Here's the drawing with two shaded views (mm, measured from the low corner). I have some questions. A direction names the side the tool comes from. Give positions to 0.01 mm unless a question says otherwise; leave off trailing zeros. Loops run counter-clockwise (first coordinate to the right, second up) from the corner with the lowest first, then second, coordinate; pieces in that order, holes last. Notation, with made-up numbers: M 38.25,-32 L 74.25,-32 A29 cw 74.25,-6 Z; hole C 31.25,3.25 d8. An arc over 180 degrees is marked long. Answer in a Markdown table with one row per item. Add a question column.
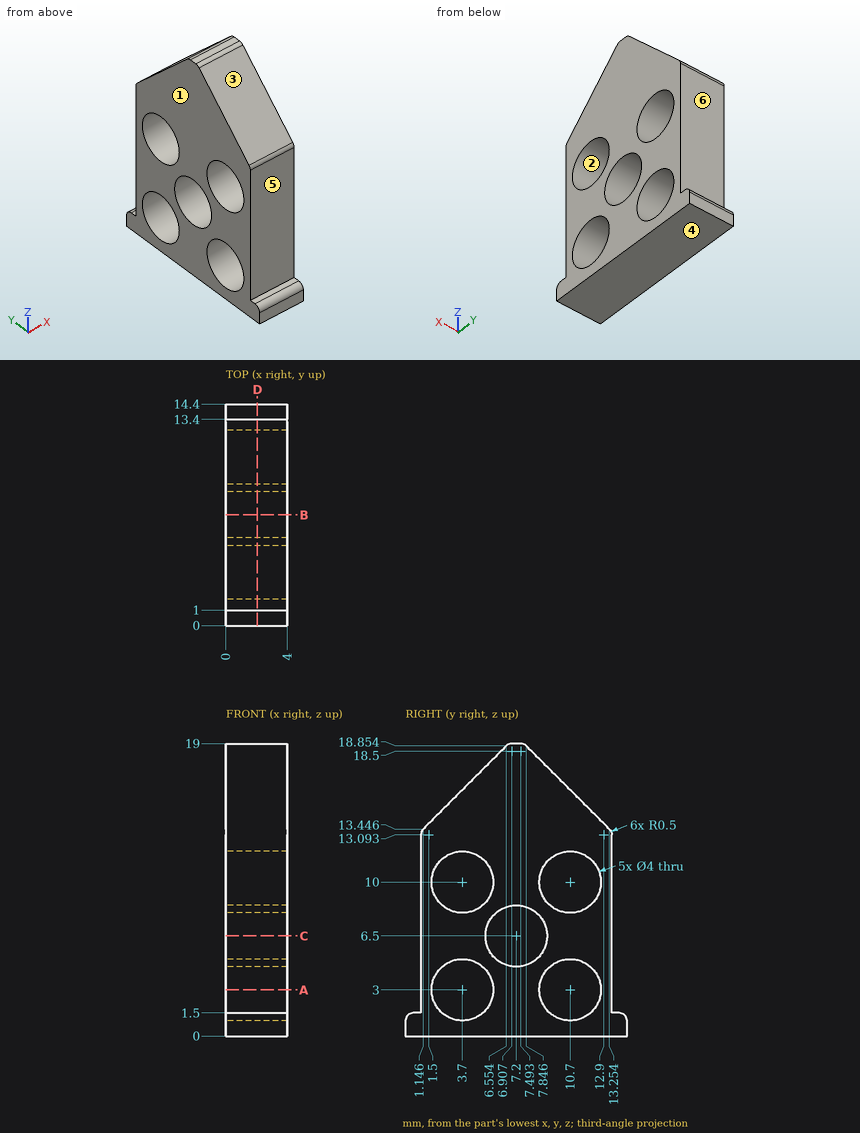
Item 1: Suppose I cut it at A-A (z = 3). List the corners of the cut face in (x, y) for me.
Item 2: If we mould it in two halves opening along Y, with no side actions, what happens to the marked faces 1, 2 and 3? For each: +Y half, -Y half, draft (parallel to the pull), parting line (faces both ways), or undercut.
Item 3: Suppose I cut it at B-B (y = 7.2). List the corners of the cut face in (x, z) for me.
Item 4: For the marked faces 4, 5 and 6, which set-ups out of +Z, -Z, +X, -X, +Y, -Y let a thin tool reach every point of the face, with its end or its side?
Item 5: I need wall thicknesses on L1, parallel to Y at x = 0.5, z = 3; L2, parallel to Y at x = 1.1, z = 6.5; L3, parallel to Y at x = 3.35, z = 11.25. Which ranges of each line are inside material? Lowest first, please.
Item 6: Suppose I cut it at D-D (x = 2.05). List the corners of the cut face in (y, z) for me.
Item 7: Suppose I cut it at C-C (z = 6.5). List the corners of the cut face in (x, y) for me, then the cut area to 3 significant figures.
Item 8: For P1, Ø3.5, axis at y = 3.7, z = 3, coming from the +X side; P2, Ø5, axis at y = 7.2, z = 6.5, coming from the +X side; P3, Ø1.5, axis at x = 2, z = 8.5, coming from the -Y side, each with a flat end and sliding along its axis, tell me the tip position at first contact or that it passes through.
Values found:
| question | item | result |
|---|---|---|
| 1 | outline | M 0,1 L 4,1 L 4,1.7 L 0,1.7 Z; M 0,5.7 L 4,5.7 L 4,8.7 L 0,8.7 Z; M 0,12.7 L 4,12.7 L 4,13.4 L 0,13.4 Z |
| 2 | face 1 | draft |
| 2 | face 2 | undercut |
| 2 | face 3 | -Y half |
| 3 | outline | M 0,0 L 4,0 L 4,4.5 L 0,4.5 Z; M 0,8.5 L 4,8.5 L 4,19 L 0,19 Z |
| 4 | face 4 | -Z, +X, -X, +Y, -Y |
| 4 | face 5 | +Z, +X, -X, -Y |
| 4 | face 6 | +Z, +X, -X, +Y |
| 5 | L1 | 1 to 1.7, 5.7 to 8.7, 12.7 to 13.4 |
| 5 | L2 | 1 to 5.2, 9.2 to 13.4 |
| 5 | L3 | 1 to 2.14, 5.26 to 9.14, 12.26 to 13.4 |
| 6 | outline | M 0,0 L 14.4,0 L 14.4,1 A0.5 ccw 13.9,1.5 L 13.4,1.5 L 13.4,13.09 A0.5 ccw 13.25,13.45 L 7.85,18.85 A0.5 ccw 7.49,19 L 6.91,19 A0.5 ccw 6.55,18.85 L 1.15,13.45 A0.5 ccw 1,13.09 L 1,1.5 L 0.5,1.5 A0.5 ccw 0,1 Z; hole C 3.7,3 d4; hole C 3.7,10 d4; hole C 7.2,6.5 d4; hole C 10.7,3 d4; hole C 10.7,10 d4 |
| 7 | outline | M 0,1 L 4,1 L 4,5.2 L 0,5.2 Z; M 0,9.2 L 4,9.2 L 4,13.4 L 0,13.4 Z |
| 7 | area | 33.6 mm² |
| 8 | P1 | through |
| 8 | P2 | x = 4 |
| 8 | P3 | y = 1 |
